Can you work these out from the model? Positions are in its coordinate system, mm. A direction names the side the tool comes from. Round coordinates to 2 decimals unless told otherwise and drop trailing zeros. Order: outer loops, then holes, each group sorted by start corner. A loop starts at its lowest first (then second) coordinate and runs counter-clockwise, first axis right, second up.
Q1. If we section it at C-C (x = 130): Please give me the cut outline in (y, z).
Q2. For faces 1 (the face through (171.577, 0, 0)), 2 (the face through (59.16, -0.69, -3.1)), which set-ups out of +Z, -Z, +X, -X, +Y, -Y let a thin tool reach every point of the face, with its end or its side?
Q3. Will these pins go through, and if not, where does the flat tip stop? P1, Ø3, axis at x = 66.5, z = 1.5, coming from the +Y side (3 decimals); P2, Ø1, axis at y = 1.5, z = 3, coming from the -X side; P3, Ø4, axis at x = 136, z = 2.5, coming from the -Y side.
Q4. If I drill on line 1 (X direction, y = 4.5, z = 1.5); line 2 (Y direction, x = 107.5, z = 1.25); line 3 (Z direction, x = 107.5, y = -1.75), over which ranges is the centre line in solid material (lowest first)?
Q5. If we section it at A-A (z = 0): Please give me the cut outline in (x, y) (3 decimals).
Q6. If we section it at D-D (x = 26.5): Please give me the cut outline in (y, z) (3 decimals).
Autodesk Inventor part; units mm, degrees
ref_plane "dia1_XY" through (0, 3.175, 0) normal (1, 0, 0) x (0, 0, -1)
ref_plane "dia1_YZ" through (0, 3.175, 0) normal (0, 0, -1) x (0, 1, 0)
ref_plane "dia1_ZX" through (0, 3.175, 0) normal (0, 1, 0) x (1, 0, 0)
sketch "Sketch_1" plane through (0, 0, 0) normal (0, 0, 1) x (1, 0, 0)
  line L0 (171.577, 0) -> (0, 0)
  line L1 (0, 0) -> (0, 3.175)
  line L2 (0, 3.175) -> (116.6876, 3.175)
  line L3 (116.6876, 3.175) -> (116.6876, 9.6203)
  line L4 (116.6876, 9.6203) -> (171.577, 9.6203)
  line L5 (171.577, 9.6203) -> (171.577, 0)
  line L6 (171.577, 0) -> (0, 0)
revolve "Revolution1" add sketch "Sketch_1" angle 360 about axis through (171.577, 0, 0) along (1, 0, 0)
sketch "Sketch_3" plane through (0, 0, 0) normal (0, 0, 1) x (1, 0, 0)
  line L0 (0, 0) -> (-12.7, 0)
  line L1 (-12.7, 0) -> (-12.7, 2.634)
  line L2 (-12.7, 2.634) -> (-12.159, 3.175)
  line L3 (-12.159, 3.175) -> (0, 3.175)
  line L4 (0, 3.175) -> (0, 0)
  line L5 (0, 0) -> (-12.7, 0)
revolve "Revolution2" add sketch "Sketch_3" angle 360 about axis through (0, 0, 0) along (1, 0, 0)
thread "Thread1"
sketch "Sketch_30" plane through (0, 0, 0) normal (0, 0, 1) x (1, 0, 0)
  line L0 (0, 0) -> (-0.254, 0)
  line L1 (-0.254, 2.921) -> (0, 2.921)
  line L2 (0, 2.921) -> (0, 3.429)
  line L3 (0, 3.429) -> (-0.254, 3.429)
  line L4 (-0.254, 3.429) -> (-0.254, 2.921)
revolve "Revolution3" cut sketch "Sketch_30" angle 360 about axis through (0, 0, 0) along (1, 0, 0)
ref_plane "dia1_XY" through (0, 3.175, 0) normal (1, 0, 0) x (0, 0, -1)
ref_plane "dia1_YZ" through (0, 3.175, 0) normal (0, 0, -1) x (0, 1, 0)
ref_plane "dia1_ZX" through (0, 3.175, 0) normal (0, 1, 0) x (1, 0, 0)
ref_plane "dia12_XY" through (0, 0, 10.9537) normal (1, 0, 0) x (0, 0, -1)
ref_plane "dia12_YZ" through (0, 0, 10.9537) normal (0, 0, -1) x (0, 1, 0)
ref_plane "dia12_ZX" through (0, 0, 10.9537) normal (0, 1, 0) x (1, 0, 0)
ref_plane "dia1r_XY" through (0, 0, 10.2235) normal (1, 0, 0) x (0, 0, -1)
ref_plane "dia1r_YZ" through (0, 0, 10.2235) normal (0, 0, -1) x (0, 1, 0)
ref_plane "dia1r_ZX" through (0, 0, 10.2235) normal (0, 1, 0) x (1, 0, 0)
ref_plane "dia2_XY" through (0, -3.175, 0) normal (1, 0, 0) x (0, 0, -1)
ref_plane "dia2_YZ" through (0, -3.175, 0) normal (0, 0, -1) x (0, 1, 0)
ref_plane "dia2_ZX" through (0, -3.175, 0) normal (0, 1, 0) x (1, 0, 0)
ref_plane "dia22_XY" through (0, 0, -10.9537) normal (1, 0, 0) x (0, 0, -1)
ref_plane "dia22_YZ" through (0, 0, -10.9537) normal (0, 0, -1) x (0, 1, 0)
ref_plane "dia22_ZX" through (0, 0, -10.9537) normal (0, 1, 0) x (1, 0, 0)
ref_plane "dia2r_XY" through (0, 0, -10.2235) normal (1, 0, 0) x (0, 0, -1)
ref_plane "dia2r_YZ" through (0, 0, -10.2235) normal (0, 0, -1) x (0, 1, 0)
ref_plane "dia2r_ZX" through (0, 0, -10.2235) normal (0, 1, 0) x (1, 0, 0)
ref_plane "rl1_XY" through (-12.7, 0, 0) normal (1, 0, 0) x (0, 0, -1)
ref_plane "rl1_YZ" through (-12.7, 0, 0) normal (0, 0, -1) x (0, 1, 0)
ref_plane "rl1_ZX" through (-12.7, 0, 0) normal (0, 1, 0) x (1, 0, 0)
ref_plane "rl2_XY" through (0, 0, 0) normal (1, 0, 0) x (0, 0, -1)
ref_plane "rl2_YZ" through (0, 0, 0) normal (0, 0, -1) x (0, 1, 0)
ref_plane "rl2_ZX" through (0, 0, 0) normal (0, 1, 0) x (1, 0, 0)
ref_plane "rod_cp_XY" through (0, 0, 0) normal (1, 0, 0) x (0, 0, -1)
ref_plane "rod_cp_YZ" through (0, 0, 0) normal (0, 0, -1) x (0, 1, 0)
ref_plane "rod_cp_ZX" through (0, 0, 0) normal (0, 1, 0) x (1, 0, 0)
ref_plane "stroke1_XY" through (0, 0, 0) normal (1, 0, 0) x (0, 0, -1)
ref_plane "stroke1_YZ" through (0, 0, 0) normal (0, 0, -1) x (0, 1, 0)
ref_plane "stroke1_ZX" through (0, 0, 0) normal (0, 1, 0) x (1, 0, 0)
ref_plane "thd1_XY" through (-12.7, 3.175, 0) normal (1, 0, 0) x (0, 0, -1)
ref_plane "thd1_YZ" through (-12.7, 3.175, 0) normal (0, 0, -1) x (0, 1, 0)
ref_plane "thd1_ZX" through (-12.7, 3.175, 0) normal (0, 1, 0) x (1, 0, 0)
ref_plane "thd2_XY" through (-12.7, -3.175, 0) normal (1, 0, 0) x (0, 0, -1)
ref_plane "thd2_YZ" through (-12.7, -3.175, 0) normal (0, 0, -1) x (0, 1, 0)
ref_plane "thd2_ZX" through (-12.7, -3.175, 0) normal (0, 1, 0) x (1, 0, 0)
ref_plane "to_rod_clevis_XY" through (-16.764, 0, 0) normal (1, 0, 0) x (0, 0, -1)
ref_plane "to_rod_clevis_YZ" through (-16.764, 0, 0) normal (0, 0, -1) x (0, 1, 0)
ref_plane "to_rod_clevis_ZX" through (-16.764, 0, 0) normal (0, 1, 0) x (1, 0, 0)
properties part number "C-043-R0000_rod"
Solution:
1. outline: circle Ø19.24 at (0, 0)
2. face 1: +Z, -Z, +X, +Y, -Y
2. face 2: -X
3. P1: stops at y = 3.175
3. P2: stops at x = -12.48
3. P3: stops at y = -9.61
4. line 1: x = 116.69 to 171.58
4. line 2: y = -2.92 to 2.92
4. line 3: z = -2.65 to 2.65
5. outline: (-12.7, -2.634) - (-12.159, -3.175) - (-0.254, -3.175) - (-0.254, -2.921) - (0, -2.921) - (0, -3.175) - (116.688, -3.175) - (116.688, -9.62) - (171.577, -9.62) - (171.577, 9.62) - (116.688, 9.62) - (116.688, 3.175) - (0, 3.175) - (0, 2.921) - (-0.254, 2.921) - (-0.254, 3.175) - (-12.159, 3.175) - (-12.7, 2.634) - close
6. outline: circle Ø6.35 at (0, 0)
